Part model, mm, in its own coordinate system. A direction names the side the tool comes from. Give positions to 0.01 mm unless a question says otherwise; leave off trailing zeros. Order: outer loops, then holes, each group sorted by start corner. A loop starts at its lowest first (then second) coordinate and runs counter-clockwise, first axis right, second up. Notation, with made-up numbers: M 61.5,46.25 L 89.5,46.25 A18 cw 89.5,71.25 Z; hole C 24,42 d3. An arc over 180 degrees is marked long. Write each question's results on one line, items separated by ' | '. Start each with the question number.
from build123d import *

# Parameters (mm, degrees)
BOSS_EXTRUDE1_DEPTH = 10
SKETCH2_R           = 5
CUT_EXTRUDE1_DEPTH  = 26
FILLET4_R           = 10
FILLET5_R           = 10
FILLET6_R           = 10
FILLET7_R           = 10
CUT_EXTRUDE2_DEPTH  = 26
FILLET9_R           = 10
CUT_EXTRUDE3_DEPTH  = 31
CUT_EXTRUDE5_DEPTH  = 32
FILLET10_R          = 10
FILLET11_R          = 10
FILLET12_R          = 10
FILLET13_R          = 10


with BuildPart() as part:
    # Sketch1 → Boss-Extrude1 (new body)
    with BuildSketch(Plane(origin=(0, 0, 0), x_dir=(1, 0, 0), z_dir=(0, 1, 0))):
        Polygon((0, 0), (-130, 0), (-130, 50), (-80, 50), (-80, 80), (-50, 80), (-50, 50), (0, 50), align=None)
    extrude(amount=BOSS_EXTRUDE1_DEPTH)

    # Sketch2 → Cut-Extrude1 (cut)
    with BuildSketch(Plane(origin=(0, 10, 0), x_dir=(1, 0, 0), z_dir=(0, 1, 0))):
        with Locations(Location((-95, 25, 0), (0, 0, 270))):
            Circle(SKETCH2_R)
        with Locations(Location((-35, 25, 0), (0, 0, 270))):
            Circle(SKETCH2_R)
    extrude(amount=-CUT_EXTRUDE1_DEPTH, mode=Mode.SUBTRACT)

    # Fillet4
    fillet4_edges = [part.edges().sort_by_distance(p)[0] for p in [
        (-130, 5, -50),
        (-80, 5, -80),
    ]]
    fillet(fillet4_edges, radius=FILLET4_R)

    # Fillet5
    fillet5_edges = [part.edges().sort_by_distance(p)[0] for p in [
        (-50, 5, -80),
    ]]
    fillet(fillet5_edges, radius=FILLET5_R)

    # Fillet6
    fillet6_edges = [part.edges().sort_by_distance(p)[0] for p in [
        (0, 5, -50),
    ]]
    fillet(fillet6_edges, radius=FILLET6_R)

    # Fillet7
    fillet7_edges = [part.edges().sort_by_distance(p)[0] for p in [
        (0, 5, 0),
    ]]
    fillet(fillet7_edges, radius=FILLET7_R)

    # Sketch3 → Cut-Extrude2 (cut)
    with BuildSketch(Plane(origin=(0, 10, 0), x_dir=(1, 0, 0), z_dir=(0, 1, 0))):
        with BuildLine():
            Line((-70.493261523, 55), (-70.493261523, 25))
            ThreePointArc((-70.493261523, 25), (-65.493261523, 20), (-60.493261523, 25))
            Line((-60.493261523, 25), (-60.493261523, 55))
            ThreePointArc((-60.493261523, 55), (-65.493261523, 60), (-70.493261523, 55))
        make_face()
    extrude(amount=-CUT_EXTRUDE2_DEPTH, mode=Mode.SUBTRACT)

    # Fillet9
    fillet9_edges = [part.edges().sort_by_distance(p)[0] for p in [
        (-130, 5, 0),
    ]]
    fillet(fillet9_edges, radius=FILLET9_R)

    # Sketch5 → Cut-Extrude3 (cut)
    with BuildSketch(Plane(origin=(0, 10, 0), x_dir=(1, 0, 0), z_dir=(0, 1, 0))):
        with BuildLine():
            Line((-115, 0), (-115, 50))
            Line((-115, 50), (-120, 50))
            ThreePointArc((-120, 50), (-127.071067812, 47.071067812), (-130, 40))
            Line((-130, 40), (-130, 10))
            ThreePointArc((-130, 10), (-127.071067812, 2.928932188), (-120, 0))
            Line((-120, 0), (-115, 0))
        make_face()
    extrude(amount=-CUT_EXTRUDE3_DEPTH, mode=Mode.SUBTRACT)

    # Sketch6 → Cut-Extrude5 (cut)
    with BuildSketch(Plane(origin=(0, 10, 0), x_dir=(1, 0, 0), z_dir=(0, 1, 0))):
        with BuildLine():
            Line((-10, 50), (-15, 50))
            Line((-15, 50), (-15, 0))
            Line((-15, 0), (-10, 0))
            ThreePointArc((-10, 0), (-2.928932188, 2.928932188), (0, 10))
            Line((0, 10), (0, 40))
            ThreePointArc((0, 40), (-2.928932188, 47.071067812), (-10, 50))
        make_face()
    extrude(amount=-CUT_EXTRUDE5_DEPTH, mode=Mode.SUBTRACT)

    # Fillet10
    fillet10_edges = [part.edges().sort_by_distance(p)[0] for p in [
        (-15, 5, -50),
    ]]
    fillet(fillet10_edges, radius=FILLET10_R)

    # Fillet11
    fillet11_edges = [part.edges().sort_by_distance(p)[0] for p in [
        (-115, 5, -50),
    ]]
    fillet(fillet11_edges, radius=FILLET11_R)

    # Fillet12
    fillet12_edges = [part.edges().sort_by_distance(p)[0] for p in [
        (-15, 5, 0),
    ]]
    fillet(fillet12_edges, radius=FILLET12_R)

    # Fillet13
    fillet13_edges = [part.edges().sort_by_distance(p)[0] for p in [
        (-115, 5, 0),
    ]]
    fillet(fillet13_edges, radius=FILLET13_R)


solid = part.part
(1) Saw through at A-A on z = -37. Give the cut face in (x, y).
(2) Tool access for faces 4 (the flat face through (-70.493, 5, -40)), 5 (the flat face through (-80, 5, -60)), 6 (the flat face through (-50, 5, -60)), 7 (the flat face through (-65, 5, -80)): list every direction of +Z, -Z, +X, -X, +Y, -Y with a clear straight run to the whole face (end or side of a thin tool).
(3) Probe L1, parallel to X at y = 6.75, z = -25; L2, parallel to X at y = 8.75, z = -40.5; L3, parallel to X at y = 2, z = -54. List the from-to ranges inside material, lowest first.
(4) Drop flat-ended pins along their axis: P1, Ø5, axis at y = 3.5, z = -45, coming from the -X side; P2, Ø3, axis at x = -41.5, y = 5, coming from the -Z side; P3, Ø3, axis at y = 4, z = -62, coming from the -X side; P4, Ø13, axis at x = -95, z = -25, coming from the -Y side. Give the stop position or say it passes through.
(5) Saw through at B-B on x = -95. Give the cut face in (y, z).
(6) Pull direction Z, two halves, no side cores. Call faces 1 (the flat face through (-115, 5, -25)), 2 (the cylindrical face through (-112.15, 4.93, -46.99)), 3 (the cylindrical face through (-65.4, 5.1, -60)): +Z half, -Z half, draft (parallel to the pull), parting line (faces both ways), or undercut.
(7) Saw through at D-D on x = -84. Give the cut face in (y, z), plus the area to 3 significant figures.
(8) Saw through at C-C on y = 8.25. Give the cut face in (x, z), plus the area to 3 significant figures.
Taken from the geometry:
1) outline: M -115,0 L -70.49,0 L -70.49,10 L -115,10 Z; M -60.49,0 L -15,0 L -15,10 L -60.49,10 Z
2) face 4: +Y, -Y | face 5: -Z, -X, +Y, -Y | face 6: -Z, +X, +Y, -Y | face 7: -Z, +X, -X, +Y, -Y
3) L1: x = -115 to -100, -90 to -70.49, -60.49 to -40, -30 to -15 | L2: x = -114.99 to -70.49, -60.49 to -15.01 | L3: x = -80 to -70.49, -60.49 to -50
4) P1: stops at x = -114.68 | P2: stops at z = -50 | P3: stops at x = -80 | P4: stops at y = 0
5) outline: M 0,-50 L 10,-50 L 10,-30 L 0,-30 Z; M 0,-20 L 10,-20 L 10,0 L 0,0 Z
6) face 1: draft | face 2: -Z half | face 3: undercut
7) outline: M 0,-50 L 10,-50 L 10,0 L 0,0 Z | area: 500 mm²
8) outline: M -115,-40 A10 ccw -105,-50 L -80,-50 L -80,-70 A10 ccw -70,-80 L -60,-80 A10 ccw -50,-70 L -50,-50 L -25,-50 A10 ccw -15,-40 L -15,-10 A10 ccw -25,0 L -105,0 A10 ccw -115,-10 Z; hole C -95,-25 d10; hole M -70.49,-55 A5 ccw -60.49,-55 L -60.49,-25 A5 ccw -70.49,-25 Z; hole C -35,-25 d10 | area: 5,240 mm²
